```python
from build123d import *

# Parameters (mm, degrees)
SKETCH2_R               = 2.4
BOSS_EXTRUDE1_DEPTH     = 2
SKETCH3_R               = 3.1
BOSS_EXTRUDE2_DEPTH     = 1
SKETCH4_R               = 2.4
BOSS_EXTRUDE3_DEPTH     = 6
SKETCH5_R               = 3.1
BOSS_EXTRUDE4_DEPTH     = 1
CUT_EXTRUDE1_DEPTH      = 11.918791142
CUT_EXTRUDE1_DEPTH_BACK = 11.918791142
SKETCH7_R               = 0.25
CUT_EXTRUDE2_DEPTH      = 0.2
FILLET1_R               = 0.05
FILLET2_R               = 0.05
CUT_EXTRUDE3_DEPTH      = 11.918791142
CUT_EXTRUDE3_DEPTH_BACK = 11.918791142
SKETCH9_R               = 2.15


with BuildPart() as part:
    # Sketch2 → Boss-Extrude1 (new body)
    with BuildSketch(Plane(origin=(0, 0, 0), x_dir=(1, 0, 0), z_dir=(0, 1, 0))):
        with Locations(Location((0, 0, 0), (0, 0, 270))):
            Circle(SKETCH2_R)
    extrude(amount=BOSS_EXTRUDE1_DEPTH)

    # Sketch3 → Boss-Extrude2 (add)
    with BuildSketch(Plane(origin=(0, 2, 0), x_dir=(1, 0, 0), z_dir=(0, 1, 0))):
        with Locations(Location((0, 0, 0), (0, 0, 270))):
            Circle(SKETCH3_R)
    extrude(amount=BOSS_EXTRUDE2_DEPTH)

    # Sketch4 → Boss-Extrude3 (add)
    with BuildSketch(Plane(origin=(0, 3, 0), x_dir=(1, 0, 0), z_dir=(0, 1, 0))):
        with Locations(Location((0, 0, 0), (0, 0, 270))):
            Circle(SKETCH4_R)
    extrude(amount=BOSS_EXTRUDE3_DEPTH)

    # Sketch5 → Boss-Extrude4 (add)
    with BuildSketch(Plane(origin=(0, 9, 0), x_dir=(1, 0, 0), z_dir=(0, 1, 0))):
        with Locations(Location((0, 0, 0), (0, 0, 270))):
            Circle(SKETCH5_R)
    extrude(amount=BOSS_EXTRUDE4_DEPTH)

    # Sketch6 → Cut-Extrude1 (cut, two sides: drawn at the far end of the back side and taken through both)
    with BuildSketch(Plane.XY.offset(-CUT_EXTRUDE1_DEPTH_BACK)):
        with BuildLine():
            Line((0.5, 10), (0.5, 8))
            ThreePointArc((0.5, 8), (0, 7.5), (-0.5, 8))
            Line((-0.5, 8), (-0.5, 10))
            ThreePointArc((-0.5, 10), (0, 10.5), (0.5, 10))
        make_face()
    extrude(amount=CUT_EXTRUDE1_DEPTH + CUT_EXTRUDE1_DEPTH_BACK, mode=Mode.SUBTRACT)

    # Sketch7 → Cut-Extrude2 (cut)
    with BuildSketch(Plane(origin=(2.4, 0, 0), x_dir=(0, 0, -1), z_dir=(1, 0, 0))):
        with Locations((0, 7.248136305)):
            Circle(SKETCH7_R)
        with Locations((0, 3.994273363)):
            Circle(SKETCH7_R)
    extrude(amount=-CUT_EXTRUDE2_DEPTH, mode=Mode.SUBTRACT)

    # Fillet1
    fillet1_edges = [part.edges().sort_by_distance(p)[0] for p in [
        (2.386943652, 7.248136305, 0.25),
    ]]
    fillet(fillet1_edges, radius=FILLET1_R)

    # Fillet2
    fillet2_edges = [part.edges().sort_by_distance(p)[0] for p in [
        (2.386943652, 3.994273363, 0.25),
    ]]
    fillet(fillet2_edges, radius=FILLET2_R)

    # Sketch9 → Cut-Extrude3 (cut, two sides: drawn at the far end of the back side and taken through both)
    with BuildSketch(Plane(origin=(0, 0, 0), x_dir=(-1, 0, 0), z_dir=(0, -1, 0)).offset(-CUT_EXTRUDE3_DEPTH_BACK)):
        with Locations(Location((0, 0, 0), (0, 0, 103.447727045))):
            Circle(SKETCH9_R)
    extrude(amount=CUT_EXTRUDE3_DEPTH + CUT_EXTRUDE3_DEPTH_BACK, mode=Mode.SUBTRACT)


solid = part.part
```
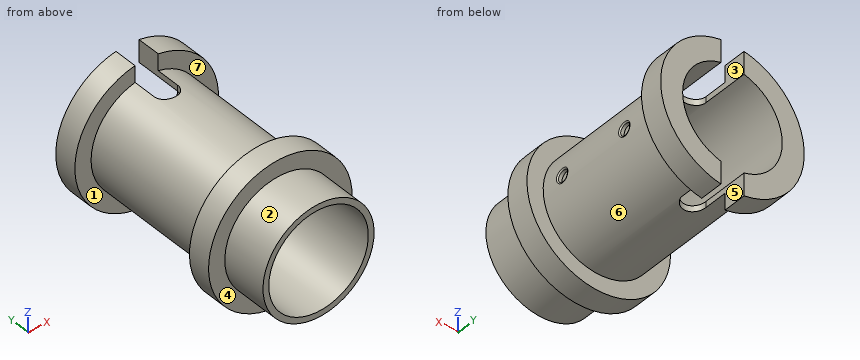
For this review, take the finished solid that the model builds, in its own axes (mm). Face numbers are marked on the shaded views. A direction names the side the tool comes from. Coordinates: 2 decimals unless noted, no trailing zeros. Write each loop counter-clockwise with the first axis right and the second up, starting at its lowest first coordinate (ties: lowest second). Pieces come first, ordered by that corner, then holes.
(1) Add section A-A on z = -1.25. Give the boundary of the cut face in (x, y), then the cut area to 3 significant figures.
(2) Add section C-C on y = 8.75. Give the boundary of the cut face in (x, z), then the cut area to 3 significant figures.
(3) The part is to be moulded in two halves that separate along Y. For the marked faces 4, 5, 6 and 7, say which applies: +Y half, -Y half, draft (parallel to the pull), parting line (faces both ways), or undercut.
(4) Tool access review of the marked faces 1, 2 and 3: name each direction out of +Z, -Z, +X, -X, +Y, -Y from which nothing blocks a thin tool from reaching the whole face with its end or side.
(5) Wall thickness on probe 1 along Y at (x, z) = (2.3, 0); probe 2 along Y at (x, z) = (2.75, -1); probe 3 along X at (y, z) = (6.5, 0): over which ranges is each line inside the solid? List them lowest first.
(6) For pin 1 Ø2 at (y, z) = (7, -2) entering from -X; pin 2 Ø3 at (x, y) = (0, 7.5) entering from -Z; pin 3 Ø0.5 at (y, z) = (9, 2.5) entering from -X, all flat-tipped, find the tip position at first contact; note any pin that passes through.
(7) Add section D-D on z = 1.75. Give the boundary of the cut face in (x, y).
(8) Add section B-B on x = 0. Give the boundary of the cut face in (y, z), then the cut area to 3 significant figures.
Answer sheet:
1. outline: (-2.84, 2) - (-2.05, 2) - (-2.05, 0) - (-1.75, 0) - (-1.75, 10) - (-2.84, 10) - (-2.84, 9) - (-2.05, 9) - (-2.05, 3) - (-2.84, 3) - close; (1.75, 0) - (2.05, 0) - (2.05, 2) - (2.84, 2) - (2.84, 3) - (2.05, 3) - (2.05, 9) - (2.84, 9) - (2.84, 10) - (1.75, 10) - close
1. area: 9.14 mm2
2. outline: (-0.5, -2.35) - (-0.5, -2.09) arc R2.15 cw to (-0.5, 2.09) - (-0.5, 2.35) arc R2.4 ccw to start; (0.5, -2.35) arc R2.4 ccw to (0.5, 2.35) - (0.5, 2.09) arc R2.15 cw to (0.5, -2.09) - close
2. area: 3.07 mm2
3. face 4: -Y half
3. face 5: draft
3. face 6: undercut
3. face 7: undercut
4. face 1: -X
4. face 2: -Y
4. face 3: +Z, -Z, +Y
5. probe 1: y = 0 to 3.74, 4.24 to 7, 7.5 to 10
5. probe 2: y = 2 to 3, 9 to 10
5. probe 3: x = -2.4 to -2.15, 2.15 to 2.4
6. pin 1: stops at x = -2.18
6. pin 2: stops at z = -2.4
6. pin 3: stops at x = -2.13
7. outline: (-2.56, 2) - (-1.64, 2) - (-1.64, 0) - (-1.25, 0) - (-1.25, 10) - (-2.56, 10) - (-2.56, 9) - (-1.64, 9) - (-1.64, 3) - (-2.56, 3) - close; (1.25, 0) - (1.64, 0) - (1.64, 2) - (2.56, 2) - (2.56, 3) - (1.64, 3) - (1.64, 9) - (2.56, 9) - (2.56, 10) - (1.25, 10) - close
8. outline: (0, -2.4) - (2, -2.4) - (2, -3.1) - (3, -3.1) - (3, -2.4) - (7.5, -2.4) - (7.5, -2.15) - (0, -2.15) - close; (0, 2.15) - (7.5, 2.15) - (7.5, 2.4) - (3, 2.4) - (3, 3.1) - (2, 3.1) - (2, 2.4) - (0, 2.4) - close
8. area: 5.15 mm2
